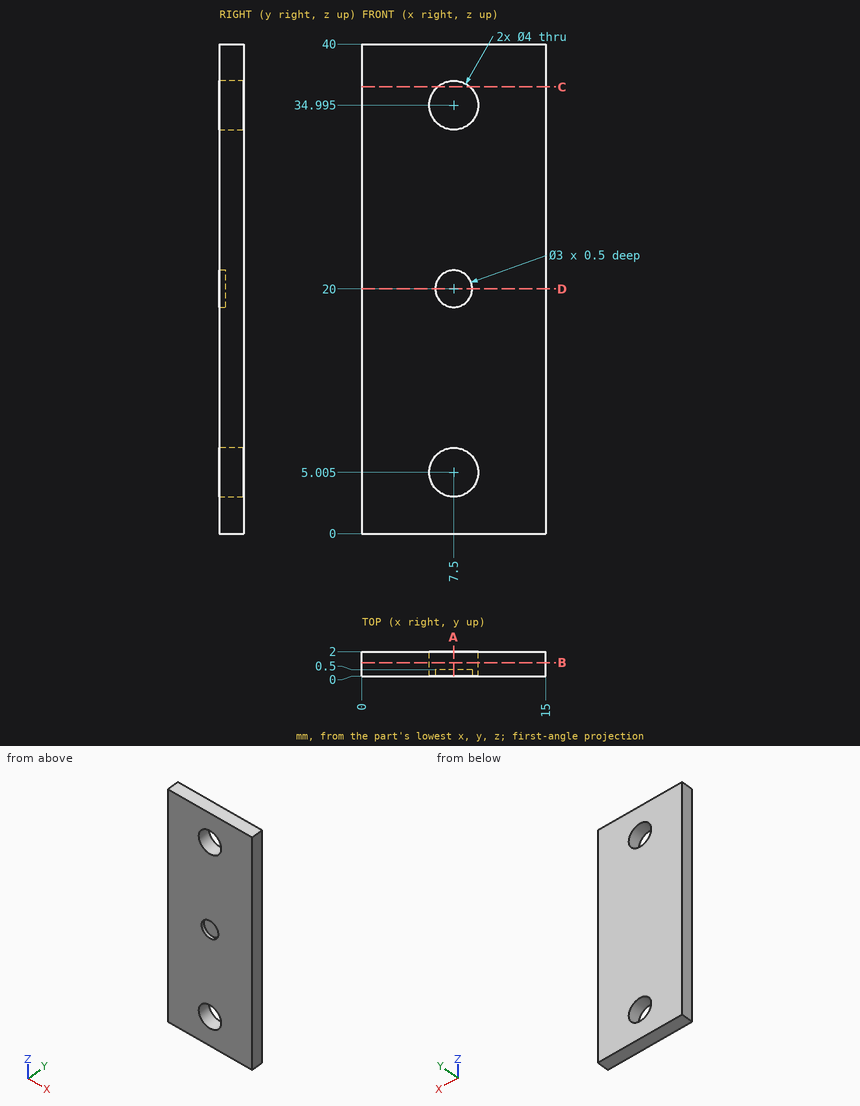
For this review, use the dimensioned drawing (mm, ordinates from the lowest corner) and the shaded views. Round coordinates to 2 decimals unless told otherwise and drop trailing zeros. Order: outer loops, then holes, each group sorted by start corner. A loop starts at its lowest first (then second) coordinate and runs counter-clockwise, first axis right, second up. Notation, with made-up numbers: M 20.5,-7.75 L 58.5,-7.75 A20 cw 58.5,5.25 Z; hole C 12.5,22 d10. An arc over 180 degrees is marked long. Use a Markdown table: item, result. Add a question column.
Item 1: Add section A-A, the plane x = 7.5. Give the boundary of the cut face in (y, z) (1 decimal).
Item 2: Add section B-B, the plane y = 1.1. Give the boundary of the cut face in (x, z) (1 decimal), then the cut area to 3 significant figures.
Item 3: To check wall thickness, follow line 1 along X through (y, z) = (0.3, 20); line 2 along X through (y, z) = (0.15, 35); line 3 along Z through (x, y) = (6, 1.75) (1 decimal). State the ranges of each line that lie inside material, in increasing order.
Item 4: Add section C-C, the plane z = 36.5. Give the boundary of the cut face in (x, y).
Item 5: Add section D-D, the plane z = 20. Give the boundary of the cut face in (x, y).
Item 6: Insertion check: pin 1 (0.9 mm diameter, centred on x = 8, z = 20, fed in from -Y); pin 2 (3.5 mm diameter, centred on x = 7.5, z = 5, fed in from +Y); pin 3 (5 mm diameter, centred on x = 7.5, z = 35, fed in from -Y). Each pin has a flat end and moves straight along its axis. Give the tip position at first contact, or say it passes through.
Geometry results:
| question | item | result |
|---|---|---|
| 1 | outline | M 0,0 L 2,0 L 2,3 L 0,3 Z; M 0,7 L 2,7 L 2,33 L 0,33 L 0,21.5 L 0.5,21.5 L 0.5,18.5 L 0,18.5 Z; M 0,37 L 2,37 L 2,40 L 0,40 Z |
| 2 | outline | M 0,0 L 15,0 L 15,40 L 0,40 Z; hole C 7.5,5 d4; hole C 7.5,35 d4 |
| 2 | area | 575 mm² |
| 3 | line 1 | x = 0 to 6, 9 to 15 |
| 3 | line 2 | x = 0 to 5.5, 9.5 to 15 |
| 3 | line 3 | z = 0 to 3.7, 6.3 to 33.7, 36.3 to 40 |
| 4 | outline | M 0,0 L 6.18,0 L 6.18,2 L 0,2 Z; M 8.82,0 L 15,0 L 15,2 L 8.82,2 Z |
| 5 | outline | M 0,0 L 6,0 L 6,0.5 L 9,0.5 L 9,0 L 15,0 L 15,2 L 0,2 Z |
| 6 | pin 1 | stops at y = 0.5 |
| 6 | pin 2 | passes through |
| 6 | pin 3 | stops at y = 0 |
